Autodesk Inventor part; units mm, degrees
ref_plane "YZ Plane" through (0, 0, 0) normal (1, 0, 0) x (0, 1, 0)
ref_plane "XZ Plane" through (0, 0, 0) normal (0, 1, 0) x (-1, 0, 0)
ref_plane "XY Plane" through (0, 0, 0) normal (0, 0, 1) x (1, 0, 0)
ref_plane "Work Plane1" through (0, 0, -5.5) normal (0, 0, 1) x (1, 0, 0)
sketch "Sketch1" plane through (0, 0, -5.5) normal (0, 0, 1) x (1, 0, 0)
  line L0 (0, 197) -> (0, 0) construction
  line L1 (0, 197) -> (-20, 197) construction
  line L2 (-20, 0) -> (-20, 197) construction
  line L3 (0, 0) -> (-20, 0) construction
  line L4 (0, 0) -> (-70, 0) construction
  line L5 (-70, 0) -> (-70, -5) construction
  line L6 (0, -5) -> (-70, -5) construction
  line L7 (0, 0) -> (0, -5) construction
  line L8 (-70, 197) -> (0, 197) construction
  line L9 (0, 197) -> (0, 202) construction
  line L10 (-70, 202) -> (0, 202) construction
  line L11 (-70, 197) -> (-70, 202) construction
  line L12 (0, 0) -> (0, 197)
  line L13 (0, 0) -> (-70, 0)
  line L14 (-70, 0) -> (-70, 25)
  line L15 (-70, 25) -> (-65, 25)
  line L16 (-65, 25) -> (-65, 172)
  line L17 (-65, 172) -> (-70, 172)
  line L18 (-70, 172) -> (-70, 197)
  line L19 (-70, 197) -> (0, 197)
  line L20 (-65, 0) -> (-65, -5) construction
  dimension "d1" = 0
  dimension "d2" = 0
  dimension "d3" = 25
  dimension "d4" = 25
extrude "Extrusion1" add sketch "Sketch1" along normal blind 5
sketch "Sketch2" plane through (0, 0, -0.5) normal (0, 0, 1) x (1, 0, 0)
  point P0 (0, 0)
sketch "Sketch3" plane through (0, 0, -5.5) normal (0, 0, -1) x (-1, 0, 0)
  line L0 (0, 0) -> (0, 197) construction
  line L1 (0, 0) -> (20, 0) construction
  line L2 (20, 197) -> (20, 0) construction
  line L3 (0, 197) -> (20, 197) construction
  line L4 (10, 197) -> (10, 0) construction
  line L5 (0, 0) -> (0, 197) construction
  line L6 (0, 98.5) -> (20, 98.5) construction
  point P0 (10, 98.5)
  point P1 (10, 177)
  point P2 (10, 20)
  dimension "d7" = 20
  dimension "d8" = 20
hole "Hole1" [suppressed]
sketch "Sketch4" plane through (-65, 25, -5.5) normal (-1, 0, 0) x (0, 0, 1)
  line L0 (0, 147) -> (0, 0) construction
  line L1 (0, 0) -> (5, 0) construction
  line L2 (5, 147) -> (5, 0) construction
  line L3 (0, 147) -> (5, 147) construction
  line L4 (2.5, 0) -> (2.5, 147) construction
  line L5 (5, 147) -> (5, 0) construction
  line L6 (5, 73.5) -> (0, 73.5) construction
  point P0 (5.5, -25)
  point P1 (2.5, 73.5)
  point P2 (2.5, 127)
  point P3 (2.5, 20)
  dimension "d16" = 20
  dimension "d17" = 20
hole "Hole2" at (-65, 98.5, -3) at (-65, 152, -3) at (-65, 45, -3) direction (1, 0, 0) diameter 2.459 depth 8.8 tip angle 118
sketch "Sketch5" plane through (0, 0, -0.5) normal (0, 0, 1) x (1, 0, 0)
  line L0 (-56.2, 46.2295) -> (-65, 46.2295) construction
  line L1 (-56.2, 43.7705) -> (-65, 43.7705) construction
  line L2 (-56.2, 99.7295) -> (-65, 99.7295) construction
  line L3 (-56.2, 97.2705) -> (-65, 97.2705) construction
  line L4 (-56.2, 153.2295) -> (-65, 153.2295) construction
  line L5 (-56.2, 150.7705) -> (-65, 150.7705) construction
  line L6 (-65, 43.7705) -> (-65, 46.2295) construction
  line L7 (-65, 43.7705) -> (-65, 46.2295) construction
  line L8 (-65, 45) -> (-57.2589, 45) construction
  line L9 (-62, 42.15) -> (-59, 42.15)
  line L10 (-59, 42.15) -> (-59, 47.85)
  line L11 (-59, 47.85) -> (-62, 47.85)
  line L12 (-62, 47.85) -> (-62, 42.15)
  line L13 (-65, 150.7705) -> (-65, 153.2295) construction
  line L14 (-65, 150.7705) -> (-65, 153.2295) construction
  line L15 (-65, 152) -> (-56.2589, 152) construction
  line L16 (-62, 149.15) -> (-59, 149.15)
  line L17 (-59, 149.15) -> (-59, 154.85)
  line L18 (-59, 154.85) -> (-62, 154.85)
  line L19 (-62, 154.85) -> (-62, 149.15)
  line L20 (-65, 97.2705) -> (-65, 99.7295) construction
  line L21 (-65, 97.2705) -> (-65, 99.7295) construction
  line L22 (-65, 98.5) -> (-54.9007, 98.5) construction
  line L23 (-62, 95.65) -> (-59, 95.65)
  line L24 (-59, 95.65) -> (-59, 101.35)
  line L25 (-59, 101.35) -> (-62, 101.35)
  line L26 (-62, 101.35) -> (-62, 95.65)
  point P0 (0, 0)
  dimension "d25" = 5.7
  dimension "d26" = 3
  dimension "d27" = 3
  dimension "d28" = 5.7
  dimension "d29" = 3
  dimension "d30" = 3
  dimension "d31" = 5.7
  dimension "d32" = 3
  dimension "d33" = 3
extrude "Extrusion2" cut sketch "Sketch5" against normal through all
sketch "Sketch6" plane through (0, 0, -5.5) normal (0, 0, -1) x (-1, 0, 0)
  line L0 (35, 87) -> (0, 87)
  arc A0 (35, 87) -> (35, 95) centre (35, 91) ccw
  line L1 (0, 95) -> (35, 95)
  line L2 (0, 95) -> (0, 87)
  line L3 (0, 0) -> (0, 197)
  line L4 (65, 153) -> (65, 110) construction
  line L5 (70, 153) -> (65, 153) construction
  line L6 (70, 110) -> (70, 153) construction
  line L7 (70, 110) -> (65, 110) construction
  line L8 (70, 131.5) -> (0, 131.5) construction
  line L9 (62, 139) -> (47, 139)
  line L10 (47, 139) -> (47, 124)
  line L11 (47, 124) -> (62, 124)
  line L12 (62, 124) -> (62, 139)
  dimension "d36" = 15
  dimension "d37" = 15
  dimension "d38" = 3
extrude "Extrusion3" [suppressed]
equation "\"d4\" = d3"
equation "\"d5\" = plate_thickness"
equation "\"plate_thickness\" = 5"
equation "\"basic_plate_offset\" = 0"
equation "\"ABS_tolerance\" = 0"
equation "\"laser_cutter_thickness\" = 0.1"
properties part number "fronts-02"
Check sheet for the modelled part. Datum: model origin and axes. Units: mm. A direction names the side the tool comes from. Round coordinates to 2 decimals unless told otherwise and drop trailing zeros. Order: outer loops, then holes, each group sorted by start corner. A loop starts at its lowest first (then second) coordinate and runs counter-clockwise, first axis right, second up. Notation, with made-up numbers: (50.5, -19) - (86.5, -19) arc R9 cw to (86.5, -10) - close; hole circle Ø10 at (-18, 13). An arc over 180 degrees is marked (long way). Write item = value, one per line.
Q1. Section check A-A (y = 118.5). Record the boundary of the cut face in (x, z).
Computed:
outline = (-65, -5.5) - (0, -5.5) - (0, -0.5) - (-65, -0.5) - close
Q2. Tool access check on faces 1 (the face through (-62, 153, -2)), 2 (the face through (-70, 184, -3)), 3 (the face through (-68, 25, -3)). Record the directions out of +Z, -Z, +X, -X, +Y, -Y that give a thin tool (end or side, any length) a straight path to the whole face; none if there is none.
Computed:
face_1 = +Z, -Z
face_2 = +Z, -Z, -X, +Y, -Y
face_3 = +Z, -Z, -X
Q3. Draft check along X on faces 4 (the face through (-35, 100, -0.5)), 5 (the face through (-62, 100, -3)), 6 (the face through (0, 97, -3)). Enter one of: pulls with the +X half, pulls with the -X half, needs draft (parallel to the pull), parting line crosses it, or undercut.
Computed:
face_4 = needs draft
face_5 = undercut
face_6 = pulls with the +X half
Q4. Go/stop test with a flat-tipped pin: pin 1 (1 mm diameter, centred on y = 139.5, z = -4.5, fed in from -X). Record where the tip stops, or that it passes through.
Computed:
pin_1 = -65
Q5. Thickness scan on line 1 along Y through (x, z) = (-62.65, -3); line 2 along X through (y, z) = (109.5, -2.45). Record the ranges inside material, lowest first.
Computed:
line_1 = 0 to 43.77, 46.23 to 97.27, 99.73 to 150.77, 153.23 to 197
line_2 = -65 to 0
